The model under review builds one solid part; all positions refer to its coordinate system, in mm. Face numbers are marked on the shaded views. A direction names the side the tool comes from. Give positions to 0.01 mm unless a question says otherwise; leave off trailing zeros. Loops run counter-clockwise (first coordinate to the right, second up) from the corner with the lowest first, then second, coordinate; pieces in that order, holes last. Notation, with made-up numbers: (73, 40.25) -> (110, 40.25) arc R35 cw to (110, 78.25) -> close; hole circle Ø8 at (44, -5). An arc over 180 degrees is marked (long way). Write each question's results on one line, items separated by ' | '. Start each with the question number.
Q1. We need section B-B (x = -54). Write out the cut boundary in (y, z).
Q2. We need section C-C (y = -40). Write out the cut boundary in (x, z).
Q3. We need section A-A (x = 1.5). Write out the cut boundary in (y, z).
Q4. We need section D-D (z = 2.25). Give the number of separate pieces and of enclosed holes in the cut face, plus the area to 3 significant figures.
Q5. Insertion check: pin 1 Ø3 at (x, y) = (-20.66, 14.05) entering from +Z; pin 2 Ø1.5 at (x, z) = (-32.5, 4.5) entering from +Y; pin 3 Ø6.5 at (x, y) = (-54.32, -19.58) entering from -Z; pin 4 Ø2 at (y, z) = (-25, 3) entering from -X. Each pin has a flat end and moves straight along its axis. Give the tip position at first contact, or say it passes through.
Q6. Wall thickness on L1, parallel to Y at x = -2, z = 2; L2, parallel to Y at x = 5, z = 3.25; L3, parallel to X at y = -17, z = 1: over which ranges is each line inside the solid? List them lowest first. Write a range as [from, to].
Q7. Machinability: for the marked faces 1, 2 and 3, which of the approach directions +Z, -Z, +X, -X, +Y, -Y give a long, thin tool a straight path to every point of the face, cutting with its end or side? Answer none if there is none.
from build123d import *

# Parameters (mm, degrees)
SKETCH1_R                 = 4
SKETCH1_R_2               = 2.527736539
BOSS_EXTRUDE1_DEPTH       = 6.35
F_5_0MM_DOWEL_SLOT1_DEPTH = 6.35
SKETCH4_R                 = 4.926776695
CUT_EXTRUDE1_DEPTH        = 3.175


# Read off the part's stored shape, not the designer's step: Ø5.0mm Dowel Slot1
with BuildPart() as part:
    # Sketch1 → Boss-Extrude1 (new body)
    with BuildSketch(Plane.XY):
        with BuildLine():
            Line((8, -57.58012907), (-20.66, -57.58012907))
            ThreePointArc((-20.66, -57.58012907), (-22.435973202, -57.254090899), (-23.980332383, -56.318496743))
            Line((-23.980332383, -56.318496743), (-58.320332383, -25.818496743))
            ThreePointArc((-58.320332383, -25.818496743), (-59.560792799, -24.12931648), (-60, -22.08012907))
            Line((-60, -22.08012907), (-60, -17.08012907))
            ThreePointArc((-60, -17.08012907), (-59.560792799, -15.03094166), (-58.320332383, -13.341761396))
            Line((-58.320332383, -13.341761396), (-23.980332383, 17.158238604))
            ThreePointArc((-23.980332383, 17.158238604), (-22.435973202, 18.09383276), (-20.66, 18.41987093))
            Line((-20.66, 18.41987093), (8, 18.41987093))
            ThreePointArc((8, 18.41987093), (9.414213562, 17.834084493), (10, 16.41987093))
            Line((10, 16.41987093), (10, -6.725270109))
            ThreePointArc((10, -6.725270109), (10.152279768, -7.490730718), (10.585929943, -8.139627163))
            Line((10.585929943, -8.139627163), (19.414070057, -16.965975896))
            ThreePointArc((19.414070057, -16.965975896), (19.847720232, -17.614872341), (20, -18.38033295))
            Line((20, -18.38033295), (20, -20.77992519))
            ThreePointArc((20, -20.77992519), (19.847720232, -21.545385798), (19.414070057, -22.194282243))
            Line((19.414070057, -22.194282243), (10.585929943, -31.020630977))
            ThreePointArc((10.585929943, -31.020630977), (10.152279768, -31.669527422), (10, -32.43498803))
            Line((10, -32.43498803), (10, -55.58012907))
            ThreePointArc((10, -55.58012907), (9.414213562, -56.994342632), (8, -57.58012907))
        make_face()
        with Locations((-20.66, -19.58012907)):
            Circle(SKETCH1_R, mode=Mode.SUBTRACT)
        with Locations((-54.318282784, -19.58012907)):
            Circle(SKETCH1_R_2, mode=Mode.SUBTRACT)
        with Locations((-20.66, 14.050414337)):
            Circle(SKETCH1_R_2, mode=Mode.SUBTRACT)
        with Locations((12.998282784, -19.58012907)):
            Circle(SKETCH1_R_2, mode=Mode.SUBTRACT)
        with Locations((-20.66, -53.238409212)):
            Circle(SKETCH1_R_2, mode=Mode.SUBTRACT)
    extrude(amount=BOSS_EXTRUDE1_DEPTH)

    # Ø5.0mm Dowel Slot1 outline → Ø5.0mm Dowel Slot1 (cut)
    with BuildSketch(Plane.XY):
        with BuildLine():
            ThreePointArc((3.85, -22.567426083), (5.629646398, -21.823233219), (6.349772676, -20.033713042))
            ThreePointArc((6.349772676, -20.033713042), (5.629646398, -18.244192864), (3.85, -17.5))
            Line((3.85, -17.5), (-3.85, -17.5))
            ThreePointArc((-3.85, -17.5), (-5.629646398, -18.244192864), (-6.349772676, -20.033713042))
            ThreePointArc((-6.349772676, -20.033713042), (-5.629646398, -21.823233219), (-3.85, -22.567426083))
            Line((-3.85, -22.567426083), (3.85, -22.567426083))
        make_face()
        with BuildLine():
            Line((-3.85, -2.5), (3.85, -2.5))
            ThreePointArc((3.85, -2.5), (6.35, 0), (3.85, 2.5))
            Line((3.85, 2.5), (-3.85, 2.5))
            ThreePointArc((-3.85, 2.5), (-6.35, 0), (-3.85, -2.5))
        make_face()
        with BuildLine():
            Line((-3.85, -42.5), (3.85, -42.5))
            ThreePointArc((3.85, -42.5), (6.35, -40), (3.85, -37.5))
            Line((3.85, -37.5), (-3.85, -37.5))
            ThreePointArc((-3.85, -37.5), (-6.35, -40), (-3.85, -42.5))
        make_face()
    extrude(amount=F_5_0MM_DOWEL_SLOT1_DEPTH, mode=Mode.SUBTRACT)

    # Sketch4 → Cut-Extrude1 (cut)
    with BuildSketch(Plane(origin=(0, 0, 0), x_dir=(-1, 0, 0), z_dir=(0, 0, -1))):
        with Locations((20.66, -19.58012907)):
            Circle(SKETCH4_R)
    extrude(amount=-CUT_EXTRUDE1_DEPTH, mode=Mode.SUBTRACT)


solid = part.part
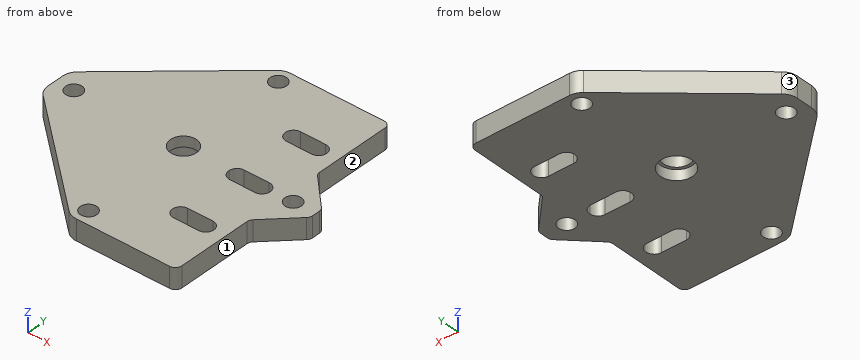
Output:
1) outline: (-29.66, 0) -> (-22.09, 0) -> (-22.09, 6.35) -> (-29.66, 6.35) -> close; (-17.07, 0) -> (-9.5, 0) -> (-9.5, 6.35) -> (-17.07, 6.35) -> close
2) outline: (-42.35, 0) -> (-6.35, 0) -> (-6.35, 6.35) -> (-42.35, 6.35) -> close; (6.35, 0) -> (10, 0) -> (10, 6.35) -> (6.35, 6.35) -> close
3) outline: (-57.58, 0) -> (-42.5, 0) -> (-42.5, 6.35) -> (-57.58, 6.35) -> close; (-37.5, 0) -> (-22.57, 0) -> (-22.57, 6.35) -> (-37.5, 6.35) -> close; (-17.5, 0) -> (-2.5, 0) -> (-2.5, 6.35) -> (-17.5, 6.35) -> close; (2.5, 0) -> (18.42, 0) -> (18.42, 6.35) -> (2.5, 6.35) -> close
4) separate pieces: 1 | enclosed holes: 8 | area: 3,880 mm2
5) pin 1: through | pin 2: y = 10.26 | pin 3: z = 0 | pin 4: x = -59.62
6) L1: [-57.58, -42.5], [-37.5, -22.57], [-17.5, -2.5], [2.5, 18.42] | L2: [-57.58, -42.22], [-37.78, -22.29], [-17.78, -2.22], [2.22, 18.42] | L3: [-60, -24.86], [-16.46, 19.45]
7) face 1: +Z, -Z, +X, -Y | face 2: +Z, -Z, +X, +Y | face 3: +Z, -Z, -X, +Y
